Autodesk Inventor part; units mm, degrees
ref_plane "YZ Plane" through (0, 0, 0) normal (1, 0, 0) x (0, 1, 0)
ref_plane "XZ Plane" through (0, 0, 0) normal (0, 1, 0) x (-1, 0, 0)
ref_plane "XY Plane" through (0, 0, 0) normal (0, 0, 1) x (1, 0, 0)
sketch "Sketch1" plane through (0, 0, 0) normal (0, 0, 1) x (1, 0, 0)
  line L0 (-165.1, 69.85) -> (165.1, 69.85)
  line L1 (165.1, 69.85) -> (165.1, -69.85)
  line L2 (165.1, -69.85) -> (-165.1, -69.85)
  line L3 (-165.1, -69.85) -> (-165.1, 69.85)
  point P0 (0, 0)
  dimension "d0" = 139.7
  dimension "d1" = 330.2
  dimension "d2" = 69.85
  dimension "d3" = 165.1
extrude "Extrusion1" add sketch "Sketch1" along normal blind 3.175
sketch "Sketch4" plane through (0, 0, 3.175) normal (0, 0, 1) x (1, 0, 0)
  line L0 (-165.1, 69.85) -> (165.1, 69.85)
  line L1 (-165.1, -69.85) -> (-165.1, 69.85)
  line L2 (165.1, -69.85) -> (-165.1, -69.85)
  line L3 (165.1, 69.85) -> (165.1, -69.85)
  line L4 (-165.1, -15.875) -> (165.1, -15.875) construction
  line L5 (0, 69.85) -> (0, -69.85) construction
  line L6 (-146.05, 69.85) -> (-146.05, -69.85) construction
  line L7 (-165.1, 66.675) -> (165.1, 66.675) construction
  point P0 (0, 0)
  point P1 (-146.05, -15.875)
  point P2 (146.05, -15.875)
  point P3 (0, -15.875)
  point P4 (-146.05, -31.75)
  point P5 (-146.05, -57.15)
  point P6 (146.05, -31.75)
  point P7 (146.05, -57.15)
  point P8 (0, 66.675)
  point P9 (-146.05, 66.675)
  point P10 (146.05, 66.675)
  dimension "d24" = 85.725
  dimension "d49" = 12.7
  dimension "d50" = 25.4
  dimension "d90" = 3.175
  dimension "d92" = 146.05
hole "Hole3" at (-146.05, -15.875, 3.175) at (146.05, -15.875, 3.175) at (0, -15.875, 3.175) at (-146.05, -31.75, 3.175) at (-146.05, -57.15, 3.175) at (146.05, -31.75, 3.175) at (146.05, -57.15, 3.175) at (-146.05, 66.675, 3.175) at (146.05, 66.675, 3.175) at (0, 66.675, 3.175) direction (0, 0, -1) diameter 3.81 end through all countersink diameter 7.0866 countersink angle 82
sketch "Sketch7" plane through (0, 0, 3.175) normal (0, 0, 1) x (1, 0, 0)
  line L0 (0, -97.79) -> (0, 97.79) construction
  line L1 (-165.1, 69.85) -> (165.1, 69.85)
  point P0 (0, 0)
  point P1 (0, 12.7)
  dimension "d51" = 57.15
hole "Hole5" at (0, 12.7, 3.175) direction (0, 0, -1) diameter 30.9563 end through all
sketch "Sketch8" plane through (0, 0, 3.175) normal (0, 0, 1) x (1, 0, 0)
  line L0 (165.1, -69.85) -> (-165.1, -69.85)
  line L1 (83.82, -69.85) -> (114.3, -69.85)
  line L2 (114.3, -69.85) -> (114.3, -48.26)
  line L3 (114.3, -48.26) -> (83.82, -48.26)
  line L4 (83.82, -48.26) -> (83.82, -69.85)
  line L5 (165.1, 69.85) -> (165.1, -69.85)
  line L6 (99.06, -48.26) -> (99.06, -69.85) construction
  point P0 (0, 0)
  point P1 (79.0575, -58.42)
  point P2 (119.0625, -58.42)
  point P3 (53.6575, -58.42)
  dimension "d59" = 30.48
  dimension "d60" = 21.59
  dimension "d61" = 50.8
  dimension "d62" = 40.005
  dimension "d63" = 11.43
  dimension "d81" = 25.4
  dimension "d82" = 11.43
extrude "Extrusion3" cut sketch "Sketch8" against normal up to next
hole "Hole6" at (79.0575, -58.42, 3.175) at (119.0625, -58.42, 3.175) direction (0, 0, -1) diameter 2.159 end through all
hole "Hole8" at (53.6575, -58.42, 3.175) direction (0, 0, -1) diameter 12.7 end through all
properties part number "J001400" material "ALUMINUM, 6061-T651"
Build history of the part. All positions in model axes, mm. Coordinates: 2 decimals unless noted, no trailing zeros. Order: outer loops, then holes, each group sorted by start corner. A loop starts at its lowest first (then second) coordinate and runs counter-clockwise, first axis right, second up. Notation, with made-up numbers: (31.5, 28) - (60.5, 28) arc R25 cw to (60.5, 41) - close; hole circle Ø8 at (80, 76). An arc over 180 degrees is marked (long way). Write each question's results on one line, items separated by ' | '. Start each with the question number.
Item 1: Mould opens along X. For faces 1 (the face through (146.65, 64.76, 1.41)), 2 (the face through (-2, 32, 3.175)) say: released by +X, released by -X, zero draft, split by the parting line, or undercut.
Item 2: Flat gauge pins, fed straight in: pin 1 (4.5 mm diameter, centred on x = 146.05, y = 66.675, fed in from +Z); pin 2 (5 mm diameter, centred on x = 0, y = 66.675, fed in from +Z); pin 3 (6 mm diameter, centred on x = -146.05, y = -31.75, fed in from -Z). Where does each tip first touch, or does it go through?
Item 3: Band-saw the part on A-A on y = 12.7. Write the cut outline in (x, z) (3 decimals).
Item 4: Band-saw the part on B-B on z = 2.45. State how many separate pieces and enclosed holes the cut face has, and give its area (3 significant figures).
Item 5: Wall check: probe 1 along X at (y, z) = (-31.75, 0.5) (3 decimals); probe 2 along Y at (x, z) = (-146.05, 0.7) (3 decimals); probe 3 along Y at (x, z) = (0, 0.8). Give the ranges that are in metal, low to high. Write a range as [from, to].
Numbers:
1) face 1: undercut | face 2: zero draft
2) pin 1: z = 1.69 | pin 2: z = 1.97 | pin 3: z = 0
3) outline: (-165.1, 0) - (-15.478, 0) - (-15.478, 3.175) - (-165.1, 3.175) - close; (15.478, 0) - (165.1, 0) - (165.1, 3.175) - (15.478, 3.175) - close
4) separate pieces: 1 | enclosed holes: 14 | area: 44,300 mm^2
5) probe 1: [-165.1, -147.955], [-144.145, 144.145], [147.955, 165.1] | probe 2: [-69.85, -59.055], [-55.245, -33.655], [-29.845, -17.78], [-13.97, 64.77], [68.58, 69.85] | probe 3: [-69.85, -17.78], [-13.97, -2.78], [28.18, 64.77], [68.58, 69.85]
